from build123d import *

# Parameters (mm, degrees)
BOSS_EXTRUDE1_DEPTH = 7.62
BOSS_EXTRUDE2_DEPTH = 57.15
FILLET1_R           = 5.08
SKETCH3_R           = 2.54
CUT_EXTRUDE1_DEPTH  = 204.09877166
SKETCH4_R           = 5.08
CUT_EXTRUDE2_DEPTH  = 183.642823634


with BuildPart() as part:
    # Sketch1 → Boss-Extrude1 (new body)
    with BuildSketch(Plane.XY):
        with BuildLine():
            Line((-28.575, 0), (-28.575, -177.8))
            Line((-28.575, -177.8), (28.575, -177.8))
            Line((28.575, -177.8), (28.575, 0))
            ThreePointArc((28.575, 0), (0, 28.575), (-28.575, 0))
        make_face()
    extrude(amount=BOSS_EXTRUDE1_DEPTH)

    # Sketch2 → Boss-Extrude2 (add, through all)
    with BuildSketch(Plane.ZY.offset(28.575)):
        with BuildLine():
            Line((0, -177.8), (30.48, -177.8))
            Line((30.48, -177.8), (30.48, -175.26))
            ThreePointArc((30.48, -175.26), (28.992102448, -171.667897552), (25.4, -170.18))
            Line((25.4, -170.18), (0, -170.18))
            Line((0, -170.18), (0, -177.8))
        make_face()
    extrude(amount=-BOSS_EXTRUDE2_DEPTH)

    # Fillet1
    fillet1_edges = [part.edges().sort_by_distance(p)[0] for p in [
        (0, -170.18, 7.62),
    ]]
    fillet(fillet1_edges, radius=FILLET1_R)

    # Sketch3 → Cut-Extrude1 (cut, through all)
    with BuildSketch(Plane(origin=(0, -170.18, 0), x_dir=(1, 0, 0), z_dir=(0, 1, 0))):
        with Locations(Location((12.7, -19.05, 0), (0, 0, 180))):
            Circle(SKETCH3_R)
        with Locations(Location((-12.7, -19.05, 0), (0, 0, 180))):
            Circle(SKETCH3_R)
    extrude(amount=-CUT_EXTRUDE1_DEPTH, mode=Mode.SUBTRACT)

    # Sketch4 → Cut-Extrude2 (cut, through all)
    with BuildSketch(Plane(origin=(0, 0, 0), x_dir=(-1, 0, 0), z_dir=(0, 0, -1))):
        Circle(SKETCH4_R)
    extrude(amount=-CUT_EXTRUDE2_DEPTH, mode=Mode.SUBTRACT)


solid = part.part
CAD build for the part. Positions are in the model's coordinates, mm. A direction names the side the tool comes from. Coordinates: 2 decimals unless noted, no trailing zeros. Order: outer loops, then holes, each group sorted by start corner. A loop starts at its lowest first (then second) coordinate and runs counter-clockwise, first axis right, second up.
Item 1: 3-axis set-ups, long thin cutter, end or side, ignore diameter. For faces 1 (the face through (0, -170.18, 19)), 2 (the face through (-28.575, -95, 7)): which of +Z, -Z, +X, -X, +Y, -Y reach the whole face in a straight line?
Check sheet entries:
face 1: +Z, +X, -X, +Y
face 2: +Z, -Z, -X, +Y, -Y
Item 2: Band-saw the part on D-D on y = -146.5. List the corners of the cut face in (x, z) (3 decimals).
Check sheet entries:
outline: (-28.575, 0) - (28.575, 0) - (28.575, 7.62) - (-28.575, 7.62) - close
Item 3: Band-saw the part on C-C on x = 18. List the corners of the cut face in (y, z), plus the area to 3 significant figures.
Check sheet entries:
outline: (-177.8, 0) - (22.19, 0) - (22.19, 7.62) - (-165.1, 7.62) arc R5.08 cw to (-170.18, 12.7) - (-170.18, 25.4) arc R5.08 ccw to (-175.26, 30.48) - (-177.8, 30.48) - close
area: 1,700 mm2
Item 4: Pin check, flat tips, straight feed: pin 1 Ø6.5 at (x, z) = (-0.5, 17.5) entering from +Y; pin 2 Ø3 at (x, y) = (-16.5, -36.5) entering from +Z. Stop position of each tip, or through.
Check sheet entries:
pin 1: stops at y = -170.18
pin 2: stops at z = 7.62
Item 5: Drill centre lines: L1, parallel to Z at x = -23, y = -144; L2, parallel to Y at x = -0.5, z = 26; L3, parallel to Y at x = 0, z = 3.25 (3 decimals). Where is each one in solid material? Low to high.
Check sheet entries:
L1: z = 0 to 7.62
L2: y = -177.8 to -170.22
L3: y = -177.8 to -5.08, 5.08 to 28.575
Item 6: Band-saw the part on A-A on z = 19.05. List the corners of the cut face in (x, y) (3 decimals), plus the area to 3 significant figures.
Check sheet entries:
outline: (-28.575, -177.8) - (-15.24, -177.8) - (-15.24, -170.18) - (-28.575, -170.18) - close; (-10.16, -177.8) - (10.16, -177.8) - (10.16, -170.18) - (-10.16, -170.18) - close; (15.24, -177.8) - (28.575, -177.8) - (28.575, -170.18) - (15.24, -170.18) - close
area: 358 mm2
Item 7: Two-plate mould, pull along Z, no slides. Class faces 3 (the face through (0, -67, 7.62)), 4 (the face through (13.25, -173.94, 16.57)), 5 (the face through (0.63, 28.57, 3.76)): +Z half, -Z half, draft (parallel to the pull), parting line (faces both ways), or undercut.
Check sheet entries:
face 3: +Z half
face 4: undercut
face 5: draft
Item 8: Band-saw the part on B-B on x = 0. List the corners of the cut face in (y, z) (3 decimals), plus the area to 3 significant figures.
Check sheet entries:
outline: (-177.8, 0) - (-5.08, 0) - (-5.08, 7.62) - (-165.1, 7.62) arc R5.08 cw to (-170.18, 12.7) - (-170.18, 25.4) arc R5.08 ccw to (-175.26, 30.48) - (-177.8, 30.48) - close; (5.08, 0) - (28.575, 0) - (28.575, 7.62) - (5.08, 7.62) - close
area: 1,670 mm2
